Here's how the part is built. I have some questions about the finished solid (model axes, mm). Face numbers are marked on the shaded views. A direction names the side the tool comes from. Round coordinates to 2 decimals unless told otherwise and drop trailing zeros. Loops run counter-clockwise (first coordinate to the right, second up) from the corner with the lowest first, then second, coordinate; pieces in that order, holes last. Notation, with made-up numbers: (-15, 22.25) -> (-9, 22.25) arc R20 ccw to (-9, 31.25) -> close; hole circle Ø11 at (58.25, -31.5). An arc over 180 degrees is marked (long way). One line per item, written item: value. Start each with the question number.
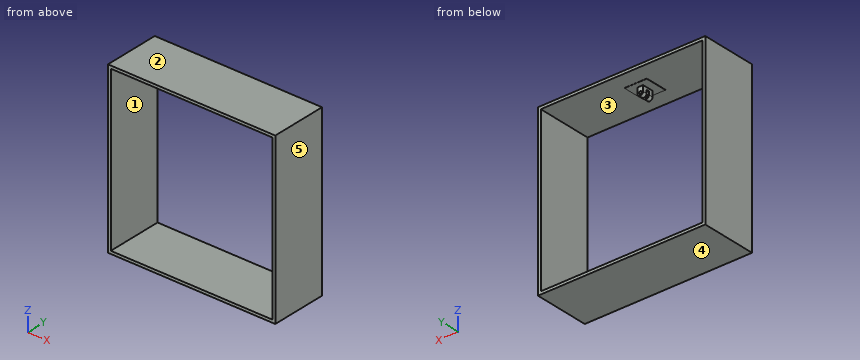
```python
from build123d import *

# Parameters (mm, degrees)
CROQUIS1_W                   = 40
CROQUIS1_H                   = 40
SALIENTE_EXTRUIR1_DEPTH      = 0.3
SALIENTE_EXTRUIR2_DEPTH      = 10
SALIENTE_EXTRUIR2_DEPTH_BACK = 10
CROQUIS2_R                   = 2.5
CORTAR_EXTRUIR1_DEPTH        = 2.5
CORTAR_EXTRUIR1_DEPTH_BACK   = 2.5
CROQUIS3_W                   = 14.056155144
CROQUIS3_H                   = 12
CROQUIS4_W                   = 300
CROQUIS4_H                   = 100
SALIENTE_EXTRUIR3_DEPTH      = 5
CROQUIS5_W                   = 300
CROQUIS5_H                   = 100
SALIENTE_EXTRUIR4_DEPTH      = 5


with BuildPart() as part:
    # Croquis1 → Saliente-Extruir1 (new body)
    with BuildSketch(Plane.XY):
        Rectangle(CROQUIS1_W, CROQUIS1_H)
    extrude(amount=SALIENTE_EXTRUIR1_DEPTH)

    # Croquis2 → Saliente-Extruir2 (add, two sides: drawn at the far end of the back side and taken through both)
    with BuildSketch(Plane(origin=(0, 0, 0), x_dir=(1, 0, 0), z_dir=(0, 1, 0)).offset(-SALIENTE_EXTRUIR2_DEPTH_BACK)):
        with BuildLine():
            Line((-5, 10), (-5, 0))
            Line((-5, 0), (5, 0))
            Line((5, 0), (5, 10))
            ThreePointArc((5, 10), (0, 15), (-5, 10))
        make_face()
        with Locations(Location((0, 10, 0), (0, 0, 270))):
            Circle(CROQUIS2_R, mode=Mode.SUBTRACT)
    extrude(amount=SALIENTE_EXTRUIR2_DEPTH + SALIENTE_EXTRUIR2_DEPTH_BACK)

    # Croquis3 → Cortar-Extruir1 (cut, two sides: drawn at the far end of the back side and taken through both)
    with BuildSketch(Plane(origin=(0, 0, 0), x_dir=(1, 0, 0), z_dir=(0, 1, 0)).offset(-CORTAR_EXTRUIR1_DEPTH_BACK)):
        with Locations((0, 10)):
            Rectangle(CROQUIS3_W, CROQUIS3_H)
    extrude(amount=CORTAR_EXTRUIR1_DEPTH + CORTAR_EXTRUIR1_DEPTH_BACK, mode=Mode.SUBTRACT)

    # Croquis4 → Saliente-Extruir3 (add)
    with BuildSketch(Plane.XY.offset(0.3)):
        Rectangle(CROQUIS4_W, CROQUIS4_H)
    saliente_extruir3 = extrude(amount=SALIENTE_EXTRUIR3_DEPTH)

    # Croquis5 → Saliente-Extruir4 (add)
    with BuildSketch(Plane(origin=(150, 0, 0), x_dir=(0, 0, -1), z_dir=(1, 0, 0))):
        with Locations((144.7, 0)):
            Rectangle(CROQUIS5_W, CROQUIS5_H)
    saliente_extruir4 = extrude(amount=-SALIENTE_EXTRUIR4_DEPTH)

    # Simetría2: Saliente-Extruir4 across plane
    add(saliente_extruir4.mirror(Plane(origin=(0, 0, 0), x_dir=(0, 0, 1), z_dir=(1, 0, 0))))

    # Simetría3: Saliente-Extruir3 across plane
    add(saliente_extruir3.mirror(Plane.XY.offset(-145)))


solid = part.part
```
Q1. I want a section at A-A on y = -28.5. Please give me the cut outline in (x, z).
Q2. If I drill on line 1 along Z through (x, y) = (0, -3); line 2 along X through (y, z) = (-4, -10); line 3 along X through (y, z) = (-22, -237), over which ranges is the centre line in solid material (lowest first)?
Q3. Which directions (+Z, -Z, +X, -X, +Y, -Y) give clear straight access to the entire face, cutting with the end or side of a thin tool? Please do the marked faces 1 and 2.
Q4. Will these pins go through, and if not, where does the flat tip stop? P1, Ø8, axis at x = -1, z = -7.5, coming from the -Y side; P2, Ø11, axis at x = 2.5, z = -11.5, coming from the +Y side.
Q5. I want a section at B-B on x = -63.5. Please give me the cut outline in (y, z).
Q6. I want a section at C-C on z = -53. Please give me the cut outline in (x, y), plus the area to 3 significant figures.
Q7. If we mould it in two halves opening along X, with no side actions, what happens to the marked faces 3, 4 and 5? For each: released by +X, released by -X, zero draft, split by the parting line, or undercut.
Answers below:
1. outline: (-150, -295.3) -> (150, -295.3) -> (150, 5.3) -> (-150, 5.3) -> close; hole (-145, -290.3) -> (145, -290.3) -> (145, 0.3) -> (-145, 0.3) -> close
2. line 1: z = -295.3 to -290.3, -15 to -12.5, -7.5 to 5.3
2. line 2: x = -150 to -145, -5 to -2.5, 2.5 to 5, 145 to 150
2. line 3: x = -150 to -145, 145 to 150
3. face 1: +Y, -Y
3. face 2: +Z, +X, -X, +Y, -Y
4. P1: stops at y = -10
4. P2: stops at y = 10
5. outline: (-50, -295.3) -> (50, -295.3) -> (50, -290.3) -> (-50, -290.3) -> close; (-50, 0.3) -> (50, 0.3) -> (50, 5.3) -> (-50, 5.3) -> close
6. outline: (-150, -50) -> (-145, -50) -> (-145, 50) -> (-150, 50) -> close; (145, -50) -> (150, -50) -> (150, 50) -> (145, 50) -> close
6. area: 1,000 mm^2
7. face 3: undercut
7. face 4: zero draft
7. face 5: released by +X
